```python
from build123d import *

# Parameters (mm, degrees)
SKETCH1_W           = 483
SKETCH1_H           = 375
BOSS_EXTRUDE1_DEPTH = 95
SKETCH2_W           = 349.080578543
SKETCH2_H           = 90
CUT_EXTRUDE1_DEPTH  = 531.118
SKETCH3_W           = 152.4
SKETCH3_H           = 100
SKETCH3_H_2         = 100.076
CUT_EXTRUDE2_DEPTH  = 531.118


with BuildPart() as part:
    # Sketch1 → Boss-Extrude1 (new body)
    with BuildSketch(Plane(origin=(0, 0, 0), x_dir=(1, 0, 0), z_dir=(0, 1, 0))):
        with Locations((25.017350158, -85.764984227)):
            Rectangle(SKETCH1_W, SKETCH1_H)
    extrude(amount=BOSS_EXTRUDE1_DEPTH)

    # Sketch2 → Cut-Extrude1 (cut)
    with BuildSketch(Plane.ZY.offset(216.482649842)):
        with Locations((85.770694956, 45)):
            Rectangle(SKETCH2_W, SKETCH2_H)
    extrude(amount=-CUT_EXTRUDE1_DEPTH, mode=Mode.SUBTRACT)

    # Sketch3 → Cut-Extrude2 (cut)
    with BuildSketch(Plane(origin=(0, 95, 0), x_dir=(1, 0, 0), z_dir=(0, 1, 0))):
        with Locations((25.071350158, -3.890984227)):
            Rectangle(SKETCH3_W, SKETCH3_H)
        with Locations((24.944350158, -167.516369345)):
            Rectangle(SKETCH3_W, SKETCH3_H_2)
    extrude(amount=-CUT_EXTRUDE2_DEPTH, mode=Mode.SUBTRACT)


solid = part.part
```
The model under review builds one solid part; all positions refer to its coordinate system, in mm. A direction names the side the tool comes from. Give positions to 0.01 mm unless a question says otherwise; leave off trailing zeros. Write each loop counter-clockwise with the first axis right and the second up, starting at its lowest first coordinate (ties: lowest second). Pieces come first, ordered by that corner, then holes.
(1) The part is to be moulded in two halves that separate along Z. For faces 3 (the flat face through (22, 47, -101.735)), 4 (the flat face through (22, 95, 83)), 5 (the flat face through (22, 90, 83)), 6 (the flat face through (22, 44, 260.311)), say which applies: released by +Z, released by -Z, zero draft, split by the parting line, or undercut.
(2) Tool access review of faces 1 (the flat face through (266.517, 93, 87)), 2 (the flat face through (22, 44, -88.77)): name each direction out of +Z, -Z, +X, -X, +Y, -Y from which nothing blocks a thin tool from reaching the whole face with its end or side.
(3) Consider section D-D, the plane x = 191. Give the boundary of the cut face in (y, z).
(4) To check wall thickness, follow L1, parallel to Z at x = 57, y = 18.5; L2, parallel to Y at x = 130.5, z = 250.5. State the ranges of each line that lie inside material, in increasing order.
(5) Consider section A-A, the plane x = -46. Give the boundary of the cut face in (y, z), and give its area (3 significant figures).
(6) Consider section C-C, the plane y = 69. Give the boundary of the cut face in (x, z).
(7) Consider section B-B, the plane z = 38.5. Give the boundary of the cut face in (x, y), and give its area (3 significant figures).
Returned:
1. face 3: released by -Z
1. face 4: zero draft
1. face 5: undercut
1. face 6: undercut
2. face 1: +Z, -Z, +X, +Y, -Y
2. face 2: +X, -X, -Y
3. outline: (0, -101.74) - (95, -101.74) - (95, 273.26) - (0, 273.26) - (0, 260.31) - (90, 260.31) - (90, -88.77) - (0, -88.77) - close
4. L1: z = -101.74 to -88.77, 260.31 to 273.26
4. L2: y = 90 to 95
5. outline: (0, -101.74) - (95, -101.74) - (95, -46.11) - (90, -46.11) - (90, -88.77) - (0, -88.77) - close; (0, 260.31) - (90, 260.31) - (90, 217.55) - (95, 217.55) - (95, 273.26) - (0, 273.26) - close; (90, 53.89) - (95, 53.89) - (95, 117.48) - (90, 117.48) - close
5. area: 3,210 mm2
6. outline: (-216.48, -101.74) - (266.52, -101.74) - (266.52, -88.77) - (-216.48, -88.77) - close; (-216.48, 260.31) - (266.52, 260.31) - (266.52, 273.26) - (-216.48, 273.26) - close
7. outline: (-216.48, 90) - (-51.13, 90) - (-51.13, 95) - (-216.48, 95) - close; (101.27, 90) - (266.52, 90) - (266.52, 95) - (101.27, 95) - close
7. area: 1,650 mm2
